from build123d import *

# Parameters (mm, degrees)
SKETCH1_R           = 8.5
BOSS_EXTRUDE1_DEPTH = 42
FILLET1_R           = 0.5


with BuildPart() as part:
    # Sketch1 → Boss-Extrude1 (new body)
    with BuildSketch(Plane(origin=(0, 0, 0), x_dir=(1, 0, 0), z_dir=(0, 1, 0))):
        Circle(SKETCH1_R)
    extrude(amount=BOSS_EXTRUDE1_DEPTH)

    # Sketch2 → M12 Tapped Hole1 (revolve, cut)
    with BuildSketch(Plane(origin=(0, 42, 0), x_dir=(0, 0, 1), z_dir=(1, 0, 0))):
        Polygon((0, 0), (0, 30.064389157), (5.1, 27), (5.1, 0), align=None)
    revolve(axis=Axis((0, 48.35, 0), (0, -1, 0)), mode=Mode.SUBTRACT)

    # Fillet1
    fillet1_edges = [part.edges().sort_by_distance(p)[0] for p in [
        (-8.5, 0, 0),
    ]]
    fillet(fillet1_edges, radius=FILLET1_R)


solid = part.part
Build history of the part. All positions in model axes, mm. Round coordinates to 2 decimals unless told otherwise and drop trailing zeros. Order: outer loops, then holes, each group sorted by start corner. A loop starts at its lowest first (then second) coordinate and runs counter-clockwise, first axis right, second up. Notation, with made-up numbers: M 59,-24.5 L 83,-24.5 A19 ccw 83,-5.5 Z; hole C 72.5,-17 d4. An arc over 180 degrees is marked long. Use CSV: the item, a comma, the result in double quotes. Start each with the question number.
(1) Cut at B-B on y = 11.5. List the corners of the cut face in (x, z), then the cut area to 3 significant figures.
(2) Mould opens along Z. For faces 1 (the face through (4.57, 20.96, -7.167)), 2 (the face through (0, 0, 0)), 3 (the face through (4.5, 28.7, 2.4)) say: +Z half, -Z half, draft (parallel to the pull), parting line (faces both ways), or undercut.
(3) Flat gauge pins, fed straight in: P1, Ø1, axis at x = -2.5, z = 3, coming from the -Y side; P2, Ø6, axis at y = 23.5, z = 4.5, coming from the -X side; P3, Ø8, axis at x = 0, z = 0, coming from the +Y side; P4, Ø2, axis at x = -5.5, y = 31, coming from the -Z side. Where does each tip first touch, or does it go through?
(4) Drill centre lines: probe 1 along X at (y, z) = (29.25, 0); probe 2 along X at (y, z) = (34.5, 4.25). Where is each one in solid material? Low to high.
(5) Cut at A-A on y = 34. List the corners of the cut face in (x, z).
Findings:
1,outline,"C 0,0 d17"
1,area,"227 mm^2"
2,face 1,"parting line"
2,face 2,"draft"
2,face 3,"undercut"
3,P1,"stops at y = 0"
3,P2,"stops at x = -8.37"
3,P3,"stops at y = 14.34"
3,P4,"stops at z = -7.21"
4,probe 1,"x = -8.5 to -5.1, 5.1 to 8.5"
4,probe 2,"x = -7.36 to -2.82, 2.82 to 7.36"
5,outline,"C 0,0 d17; hole C 0,0 d10.2"
